```python
from build123d import *

# Parameters (mm, degrees)
F0_R     = 7
F1_DEPTH = 2


with BuildPart() as f1:
    # F0 (on Top) → F1 (new body, symmetric)
    with BuildSketch(Plane.XY):
        with BuildLine():
            Line((-58.738012, 87.5), (-143, 87.5))
            Line((-143, 87.5), (-193, 37.5))
            Line((-193, 37.5), (-193, -12.5))
            Line((-193, -12.5), (-239, -39.5))
            Line((-239, -39.5), (-239, -87.5))
            Line((-239, -87.5), (239, -87.5))
            Line((239, -87.5), (239, 37.5))
            Line((239, 37.5), (189, 87.5))
            Line((189, 87.5), (50.738012, 87.5))
            ThreePointArc((50.738012, 87.5), (-4, 62), (-58.738012, 87.5))
        make_face()
        with Locations((-213.6, -54)):
            Circle(F0_R, mode=Mode.SUBTRACT)
        with Locations((213.6, -54)):
            Circle(F0_R, mode=Mode.SUBTRACT)
        with Locations((-69, 69.5)):
            Circle(F0_R, mode=Mode.SUBTRACT)
        with Locations((61, 69.5)):
            Circle(F0_R, mode=Mode.SUBTRACT)
    extrude(amount=F1_DEPTH, both=True)


solid = f1.part
```
Design review of the part built by this model. Coordinates are the model's own, in mm. Give positions to 0.01 mm unless a question says otherwise; leave off trailing zeros. Write each loop counter-clockwise with the first axis right and the second up, starting at its lowest first coordinate (ties: lowest second). Pieces come first, ordered by that corner, then holes.
(1) Mouldability with a two-part tool opening along X and no side actions: class faces 1 (the face through (-3, 1, 2)), 2 (the face through (206.607, -53.692, -0.028)), 3 (the face through (214.35, 62.15, 0.03)) as +X half, -X half, draft (parallel to the pull), parting line (faces both ways), or undercut.
Checked values:
face 1: draft
face 2: undercut
face 3: +X half
(2) Add section A-A (x = -69). Give the boundary of the cut face in (y, z).
Checked values:
outline: (-87.5, -2) - (62.5, -2) - (62.5, 2) - (-87.5, 2) - close; (76.5, -2) - (87.5, -2) - (87.5, 2) - (76.5, 2) - close
(3) Add section D-D (y = 69.5). Give the boundary of the cut face in (x, z).
Checked values:
outline: (-161, -2) - (-76, -2) - (-76, 2) - (-161, 2) - close; (-62, -2) - (-35.88, -2) - (-35.88, 2) - (-62, 2) - close; (27.88, -2) - (54, -2) - (54, 2) - (27.88, 2) - close; (68, -2) - (207, -2) - (207, 2) - (68, 2) - close
(4) Add section C-C (y = -54). Give the boundary of the cut face in (x, z).
Checked values:
outline: (-239, -2) - (-220.6, -2) - (-220.6, 2) - (-239, 2) - close; (-206.6, -2) - (206.6, -2) - (206.6, 2) - (-206.6, 2) - close; (220.6, -2) - (239, -2) - (239, 2) - (220.6, 2) - close
(5) Add section B-B (z = 0.5). Give the boundary of the cut face in (x, y), and give its area (3 significant figures).
Checked values:
outline: (-239, -87.5) - (239, -87.5) - (239, 37.5) - (189, 87.5) - (50.74, 87.5) arc R71.5 cw to (-58.74, 87.5) - (-143, 87.5) - (-193, 37.5) - (-193, -12.5) - (-239, -39.5) - close; hole circle Ø14 at (-213.6, -54); hole circle Ø14 at (-69, 69.5); hole circle Ø14 at (61, 69.5); hole circle Ø14 at (213.6, -54)
area: 73,400 mm2
(6) Clearance check with flat-ended pins moving along their axes: pin 1 Ø8.5 at (x, y) = (-69, 69.5) entering from -Z; pin 2 Ø1.5 at (y, z) = (64, -1.5) entering from -X; pin 3 Ø2 at (x, z) = (-13.5, -1) entering from +Y. State where each tip first meets the part, or that it passes through.
Checked values:
pin 1: passes through
pin 2: stops at x = -167.25
pin 3: stops at y = 62.78
(7) Wall thickness on line 1 along Y through (x, z) = (-69, -1.15); line 2 along Y through (x, z) = (213.6, -0.5); line 3 along Y through (x, z) = (-1, -0.8): over which ranges is each line inside the solid? List them lowest first.
Checked values:
line 1: y = -87.5 to 62.5, 76.5 to 87.5
line 2: y = -87.5 to -61, -47 to 62.9
line 3: y = -87.5 to 62.06
